from build123d import *

# Parameters (mm, degrees)
EXTRUDE1_DEPTH     = 2.75
CUT_EXTRUDE1_DEPTH = 15.329956996
EXTRUDE2_DEPTH     = 2.5
EXTRUDE3_DEPTH     = 1.625
SKETCH8_W          = 1
SKETCH8_H          = 0.1
EXTRUDE4_DEPTH     = 0.75
EXTRUDE5_DEPTH     = 0.5
EXTRUDE6_DEPTH     = 0.1
SKETCH11_R         = 1
SKETCH11_R_2       = 0.9
EXTRUDE7_DEPTH     = 0.5
CUT_EXTRUDE2_REACH = 24.429
SKETCH12_R         = 0.9
FILLET1_R          = 0.25


with BuildPart() as part:
    # Sketch4 → Extrude1 (new, symmetric)
    with BuildSketch(Plane(origin=(0, 0, 0), x_dir=(0, 0, -1), z_dir=(1, 0, 0))):
        with BuildLine():
            Line((-2.652797108, 12.6), (2.652797108, 12.6))
            ThreePointArc((2.652797108, 12.6), (2.769316269, 12.58857734), (2.8813989, 12.554744284))
            ThreePointArc((2.8813989, 12.554744284), (4.555213838, 11.599383852), (5.933197614, 10.251967541))
            ThreePointArc((5.933197614, 10.251967541), (6.072675346, 10.139990984), (6.247012686, 10.1))
            Line((6.247012686, 10.1), (6.247012686, 10))
            ThreePointArc((6.247012686, 10), (6.029091011, 10.04998873), (5.854743846, 10.189959426))
            ThreePointArc((5.854743846, 10.189959426), (4.494980939, 11.519559057), (2.843298601, 12.462286904))
            ThreePointArc((2.843298601, 12.462286904), (2.749896409, 12.490481117), (2.652797108, 12.5))
            Line((2.652797108, 12.5), (-2.652797108, 12.5))
            ThreePointArc((-2.652797108, 12.5), (-2.749896409, 12.490481117), (-2.843298601, 12.462286904))
            ThreePointArc((-2.843298601, 12.462286904), (-4.494980939, 11.519559057), (-5.854743846, 10.189959426))
            ThreePointArc((-5.854743846, 10.189959426), (-6.029091011, 10.04998873), (-6.247012686, 10))
            Line((-6.247012686, 10), (-6.247012686, 10.1))
            ThreePointArc((-6.247012686, 10.1), (-6.072675346, 10.139990984), (-5.933197614, 10.251967541))
            ThreePointArc((-5.933197614, 10.251967541), (-4.555213838, 11.599383852), (-2.8813989, 12.554744284))
            ThreePointArc((-2.8813989, 12.554744284), (-2.769316269, 12.58857734), (-2.652797108, 12.6))
        make_face()
    extrude(amount=EXTRUDE1_DEPTH, both=True)

    # Sketch5 → Cut-Extrude1 (cut, through all)
    with BuildSketch(Plane(origin=(0, 0, 0), x_dir=(1, 0, 0), z_dir=(0, 1, 0))):
        with BuildLine():
            Line((1.75, -3.5), (1.75, 3.5))
            ThreePointArc((1.75, 3.5), (0, 5.25), (-1.75, 3.5))
            Line((-1.75, 3.5), (-1.75, -3.5))
            ThreePointArc((-1.75, -3.5), (0, -5.25), (1.75, -3.5))
        make_face()
    extrude(amount=CUT_EXTRUDE1_DEPTH, mode=Mode.SUBTRACT)

    # Sketch6 → Extrude2 (add, symmetric)
    with BuildSketch(Plane(origin=(0, 0, 0), x_dir=(0, 0, -1), z_dir=(1, 0, 0))):
        with BuildLine():
            Line((6.247012686, 10), (7, 10))
            ThreePointArc((7, 10), (7.353553391, 9.853553391), (7.5, 9.5))
            Line((7.5, 9.5), (7.5, 8.5))
            Line((7.5, 8.5), (7.6, 8.5))
            Line((7.6, 8.5), (7.6, 9.5))
            ThreePointArc((7.6, 9.5), (7.424264069, 9.924264069), (7, 10.1))
            Line((7, 10.1), (6.247012686, 10.1))
            Line((6.247012686, 10.1), (6.247012686, 10))
        make_face()
        with BuildLine():
            Line((-7.5, 8.5), (-7.6, 8.5))
            Line((-7.6, 8.5), (-7.6, 9.5))
            ThreePointArc((-7.6, 9.5), (-7.424264069, 9.924264069), (-7, 10.1))
            Line((-7, 10.1), (-6.247012686, 10.1))
            Line((-6.247012686, 10.1), (-6.247012686, 10))
            Line((-6.247012686, 10), (-7, 10))
            ThreePointArc((-7, 10), (-7.353553391, 9.853553391), (-7.5, 9.5))
            Line((-7.5, 9.5), (-7.5, 8.5))
        make_face()
    extrude(amount=EXTRUDE2_DEPTH, both=True)

    # Sketch7 → Extrude3 (add, symmetric)
    with BuildSketch(Plane(origin=(0, 0, 0), x_dir=(0, 0, -1), z_dir=(1, 0, 0))):
        with BuildLine():
            Line((7.5, 8.5), (7.5, 7.4))
            ThreePointArc((7.5, 7.4), (7.646446609, 7.046446609), (8, 6.9))
            Line((8, 6.9), (8.75, 6.9))
            Line((8.75, 6.9), (8.75, 7))
            Line((8.75, 7), (8, 7))
            ThreePointArc((8, 7), (7.717157288, 7.117157288), (7.6, 7.4))
            Line((7.6, 7.4), (7.6, 8.5))
            Line((7.6, 8.5), (7.5, 8.5))
        make_face()
    extrude(amount=EXTRUDE3_DEPTH, both=True)

    # Sketch8 → Extrude4 (add, symmetric)
    with BuildSketch(Plane(origin=(0, 0, 0), x_dir=(0, 0, -1), z_dir=(1, 0, 0))):
        with Locations((9.25, 6.95)):
            Rectangle(SKETCH8_W, SKETCH8_H)
    extrude(amount=EXTRUDE4_DEPTH, both=True)

    # Sketch9 → Extrude5 (add, symmetric)
    with BuildSketch(Plane(origin=(0, 0, 0), x_dir=(0, 0, -1), z_dir=(1, 0, 0))):
        with BuildLine():
            Line((10.75, 7.4), (10.75, 7.9))
            Line((10.75, 7.9), (10.65, 7.9))
            Line((10.65, 7.9), (10.65, 7.4))
            ThreePointArc((10.65, 7.4), (10.532842712, 7.117157288), (10.25, 7))
            Line((10.25, 7), (9.75, 7))
            Line((9.75, 7), (9.75, 6.9))
            Line((9.75, 6.9), (10.25, 6.9))
            ThreePointArc((10.25, 6.9), (10.603553391, 7.046446609), (10.75, 7.4))
        make_face()
    extrude(amount=EXTRUDE5_DEPTH, both=True)

    # Sketch10 → Extrude6 (add)
    with BuildSketch(Plane.XY.offset(7.5)):
        with BuildLine():
            Line((-1.5, 8.5), (-1.5, 7))
            ThreePointArc((-1.5, 7), (0, 5.5), (1.5, 7))
            Line((1.5, 7), (1.5, 8.5))
            Line((1.5, 8.5), (-1.5, 8.5))
        make_face()
    extrude(amount=EXTRUDE6_DEPTH)

    # Sketch11 → Extrude7 (add)
    with BuildSketch(Plane.XY.offset(7.6)):
        with Locations(Location((0, 7, 0), (0, 0, 90))):
            Circle(SKETCH11_R)
        with Locations((0, 7)):
            Circle(SKETCH11_R_2, mode=Mode.SUBTRACT)
    extrude(amount=EXTRUDE7_DEPTH)

    # Sketch12 → Cut-Extrude2 (cut, up to next)
    with BuildSketch(Plane.XY.offset(7.6), mode=Mode.PRIVATE) as cut_extrude2_sk1:
        with Locations((0, 7)):
            Circle(SKETCH12_R)
    cut_extrude2_tool1 = extrude(cut_extrude2_sk1.sketch, amount=-CUT_EXTRUDE2_REACH, mode=Mode.PRIVATE) & part.part
    add(cut_extrude2_tool1.solids().sort_by_distance((0, 7, 7.6))[0], mode=Mode.SUBTRACT)

    # Fillet1
    fillet1_edges = [part.edges().sort_by_distance(p)[0] for p in [
        (-0.5, 7.9, -10.7),
        (0.5, 7.9, -10.7),
    ]]
    fillet(fillet1_edges, radius=FILLET1_R)


solid = part.part
Verification items for the finished model (mm, model axes). Give positions to 0.01 mm unless a question says otherwise; leave off trailing zeros. Loops run counter-clockwise (first coordinate to the right, second up) from the corner with the lowest first, then second, coordinate; pieces in that order, holes last. Notation, with made-up numbers: (-10.5, -35.75) - (13.5, -35.75) arc R24 ccw to (13.5, -3.75) - close; hole circle Ø6 at (-35.5, -23.75). An arc over 180 degrees is marked (long way). Write item = value, one per line. Start each with the question number.
Q1. Thickness scan on line 1 (Z direction, x = -2.25, y = 12). Record the ranges inside material, lowest first.
Q2. Cross-section at B-B, the plane x = 1.2. Enter the section's corners in (y, z), and give its area (3 significant figures).
Q3. Depth check by flat-ended pin: P1, Ø1.1, axis at x = 0.5, z = -9.5, coming from the -Y side; P2, Ø1.1, axis at x = 0, y = 7, coming from the +Z side; P3, Ø1, axis at y = 6, z = 6, coming from the -X side; P4, Ø1, axis at x = -1.5, z = -3, coming from the -Y side. Enter the tip coordinate at first touch or a pass-through.
Q4. Cross-section at C-C, the plane z = -4. Enter the section's corners in (x, y), and give its area (3 significant figures).
Q5. Cross-section at A-A, the plane y = 8.75. Enter the section's corners in (x, z).
Q6. Cross-section at D-D, the plane x = 0. State how many separate pieces and enclosed holes the cut face has, and give its area (3 significant figures).
Answer key:
q1.line_1 = -3.97 to -3.77, 3.77 to 3.97
q2.outline = (6.1, 7.5) - (9.5, 7.5) arc R0.5 cw to (10, 7) - (10, 6.25) arc R0.5 ccw to (10.19, 5.85) arc R7.46 cw to (11.3, 4.77) - (11.43, 4.77) arc R7.56 ccw to (10.25, 5.93) arc R0.4 cw to (10.1, 6.25) - (10.1, 7) arc R0.6 ccw to (9.5, 7.6) - (6.1, 7.6) - close; (6.9, -8.75) - (7, -8.75) - (7, -8) arc R0.4 cw to (7.4, -7.6) - (9.5, -7.6) arc R0.6 ccw to (10.1, -7) - (10.1, -6.25) arc R0.4 cw to (10.25, -5.93) arc R7.56 ccw to (11.43, -4.77) - (11.3, -4.77) arc R7.46 cw to (10.19, -5.85) arc R0.5 ccw to (10, -6.25) - (10, -7) arc R0.5 cw to (9.5, -7.5) - (7.4, -7.5) arc R0.5 ccw to (6.9, -8) - close
q2.area = 1.42 mm^2
q3.P1 = 6.9
q3.P2 = -7.5
q3.P3 = through
q3.P4 = 12.19
q4.outline = (-2.75, 11.86) - (-1.68, 11.86) - (-1.68, 11.98) - (-2.75, 11.98) - close; (1.68, 11.86) - (2.75, 11.86) - (2.75, 11.98) - (1.68, 11.98) - close
q4.area = 0.254 mm^2
q5.outline = (-2.5, -7.6) - (2.5, -7.6) - (2.5, -7.5) - (-2.5, -7.5) - close; (-2.5, 7.5) - (2.5, 7.5) - (2.5, 7.6) - (-2.5, 7.6) - close
q6.separate_pieces = 3
q6.enclosed_holes = 0
q6.area = 1.54 mm^2
